For this review, use the dimensioned drawing (mm, ordinates from the lowest corner) and the shaded views. Coordinates: 2 decimals unless noted, no trailing zeros. Loops run counter-clockwise (first coordinate to the right, second up) from the corner with the lowest first, then second, coordinate; pieces in that order, holes last. Notation, with made-up numbers: M 57,1.5 L 85,1.5 A22 cw 85,31.5 Z; hole C 38,-17.75 d10. An arc over 180 degrees is marked long. Write item = value, one per line.
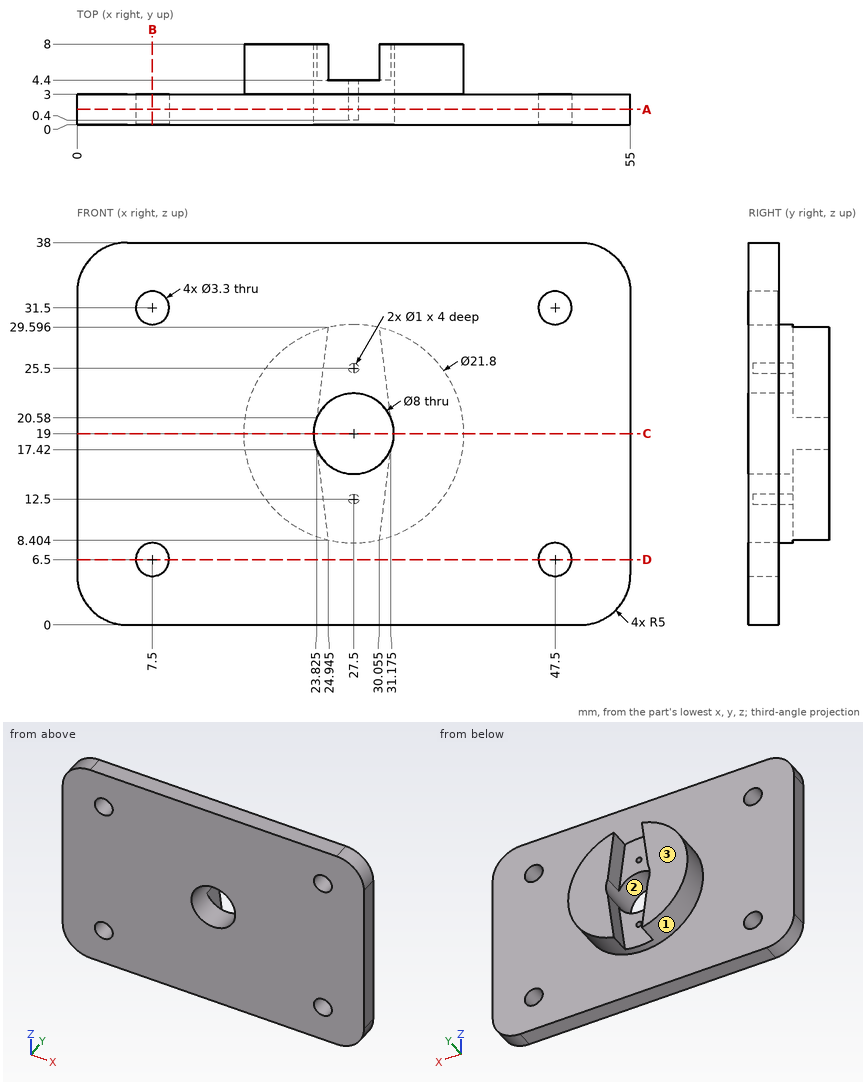
Q1. For pin 1 Ø2.5 at (x, z) = (47.5, 31.5) entering from +Y; pin 2 Ø1.1 at (x, z) = (27.5, 12.5) entering from +Y; pin 3 Ø2 at (y, z) = (5, 17.5) entering from -X, all flat-tipped, find the tip position at first contact; note any pin that passes through.
Solved:
pin_1 = through
pin_2 = 4.4
pin_3 = 16.61
Q2. Add section A-A (y = 1.5). Write out the cut boundary in (x, z).
Solved:
outline = M 0,5 A5 ccw 5,0 L 50,0 A5 ccw 55,5 L 55,33 A5 ccw 50,38 L 5,38 A5 ccw 0,33 Z; hole C 7.5,6.5 d3.3; hole C 7.5,31.5 d3.3; hole C 27.5,19 d8; hole C 27.5,12.5 d1; hole C 27.5,25.5 d1; hole C 47.5,6.5 d3.3; hole C 47.5,31.5 d3.3
Q3. Add section B-B (x = 7.5). Write out the cut boundary in (y, z).
Solved:
outline = M 0,0 L 3,0 L 3,4.85 L 0,4.85 Z; M 0,8.15 L 3,8.15 L 3,29.85 L 0,29.85 Z; M 0,33.15 L 3,33.15 L 3,38 L 0,38 Z
Q4. Add section D-D (z = 6.5). Write out the cut boundary in (x, y).
Solved:
outline = M 0,0 L 5.85,0 L 5.85,3 L 0,3 Z; M 9.15,0 L 45.85,0 L 45.85,3 L 9.15,3 Z; M 49.15,0 L 55,0 L 55,3 L 49.15,3 Z
Q5. Draft analysis for pull direction X (two halves, no side actions). For the marked faces 1, 2 and 3, state which applies: +X half, -X half, draft (parallel to the pull), parting line (faces both ways), or undercut.
Solved:
face_1 = parting line
face_2 = undercut
face_3 = draft
Q6. Add section C-C (z = 19). Write out the cut boundary in (x, y).
Solved:
outline = M 0,0 L 23.5,0 L 23.5,8 L 16.6,8 L 16.6,3 L 0,3 Z; M 31.5,0 L 55,0 L 55,3 L 38.4,3 L 38.4,8 L 31.5,8 Z
Q7. For line 1 along X through (y, z) = (1.1, 31.5); line 2 along Y through (x, z) = (11, 32); line 3 along Y through (x, z) = (24, 21), list the stretches that pass through material, from the lowest coordinate up.
Solved:
line_1 = 0 to 5.85, 9.15 to 45.85, 49.15 to 55
line_2 = 0 to 3
line_3 = 0 to 4.4
